The model under review builds one solid part; all positions refer to its coordinate system, in mm. Face numbers are marked on the shaded views. A direction names the side the tool comes from. Coordinates: 2 decimals unless noted, no trailing zeros. Loops run counter-clockwise (first coordinate to the right, second up) from the corner with the lowest first, then second, coordinate; pieces in that order, holes last. Notation, with made-up numbers: (73.25, 21.5) - (99.25, 21.5) arc R11 ccw to (99.25, 39.5) - close; hole circle Ø6 at (45.5, 61). An arc over 180 degrees is marked (long way). Use a Markdown table: item, result. Add a question column.
1) The part is to be moulded in two halves that separate along Z. For the marked faces 1, 2, 3 and 4, say which applies: pulls with the +Z half, pulls with the -Z half, needs draft (parallel to the pull), parting line crosses it, or undercut.
2) Clearance check with flat-ended pins moving along their axes: pin 1 (2 mm diameter, centred on x = -1, y = 8.5, fed in from -Z); pin 2 (2 mm diameter, centred on x = -1.5, y = 3.5, fed in from +Z); pin 3 (2 mm diameter, centred on y = 5, z = 0.5, fed in from -X). State where each tip first meets the part, or that it passes through.
3) Add section A-A, the plane x = 1.65. Give the boundary of the cut face in (y, z).
4) Add section B-B, the plane y = 5. Give the boundary of the cut face in (x, z), and give its area (3 significant figures).
5) For the marked faces 5, 6 and 7, list the 3-axis set-ups (+Z, -Z, +X, -X, +Y, -Y) from which the entire face can be reached by the end or side of a thin tool; tool diameter is ignored.
6) To check wall thickness, follow L1, parallel to Y at x = 1.6, z = 0.3; L2, parallel to X at y = 5, z = 1.3; L3, parallel to X at y = 6.75, z = 0.1. State the ranges of each line that lie inside material, in increasing order. Write a range as [from, to].
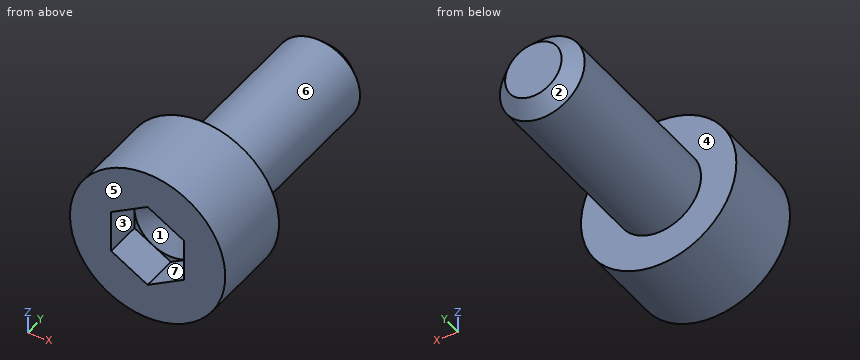
Autodesk Inventor part; units mm, degrees
ref_plane "YZ Plane" through (0, 0, 0) normal (1, 0, 0) x (0, 1, 0)
ref_plane "XZ Plane" through (0, 0, 0) normal (0, 1, 0) x (-1, 0, 0)
ref_plane "XY Plane" through (0, 0, 0) normal (0, 0, 1) x (1, 0, 0)
sketch "Boceto1" plane through (0, 0, 0) normal (0, 1, 0) x (-1, 0, 0)
  circle A0 centre (0, 0) radius 2.75
  dimension "d0" = 5.5
extrude "Extrusión1" add sketch "Boceto1" along normal blind 3
sketch "Boceto2" plane through (0, 0, 0) normal (0, -1, 0) x (1, 0, 0)
  point P0 (0, 0)
  point P1 (0, 0)
hole "Agujero1" at (0, 0, 0) direction (0, 1, 0) diameter 2.58 depth 1.3 tip angle 118
sketch "Boceto3" plane through (0, 0, 0) normal (0, -1, 0) x (1, 0, 0)
  circle A0 centre (0, 0) radius 1.29
  line L0 (0, 1.4896) -> (1.29, 0.7448)
  line L1 (1.29, 0.7448) -> (1.29, -0.7448)
  line L2 (1.29, -0.7448) -> (0, -1.4896)
  line L3 (0, -1.4896) -> (-1.29, -0.7448)
  line L4 (-1.29, -0.7448) -> (-1.29, 0.7448)
  line L5 (-1.29, 0.7448) -> (0, 1.4896)
extrude "Extrusión2" cut sketch "Boceto3" against normal blind 1.3
sketch "Boceto4" plane through (0, 3, 0) normal (0, 1, 0) x (1, 0, 0)
  circle A0 centre (0, 0) radius 1.5
  dimension "d12" = 3
extrude "Extrusión3" add sketch "Boceto4" along normal blind 7
thread "Rosca1"
chamfer "Chaflán1" distance 0.5 angle 45 1 edges at (-1.5, 10, 0)
properties part number "TornilloM3" material "Hierro, gris"
From the geometry:
| question | item | result |
|---|---|---|
| 1 | face 1 | undercut |
| 1 | face 2 | parting line crosses it |
| 1 | face 3 | undercut |
| 1 | face 4 | needs draft |
| 2 | pin 1 | stops at z = -1.5 |
| 2 | pin 2 | stops at z = 2.68 |
| 2 | pin 3 | stops at x = -1.5 |
| 3 | outline | (0, -2.2) - (3, -2.2) - (3, 2.2) - (0, 2.2) - close |
| 4 | outline | circle Ø3 at (0, 0) |
| 4 | area | 7.07 mm^2 |
| 5 | face 5 | +Z, -Z, +X, -X, -Y |
| 5 | face 6 | +Y |
| 5 | face 7 | -Y |
| 6 | L1 | y = [0, 3] |
| 6 | L2 | x = [-0.75, 0.75] |
| 6 | L3 | x = [-1.5, 1.5] |
